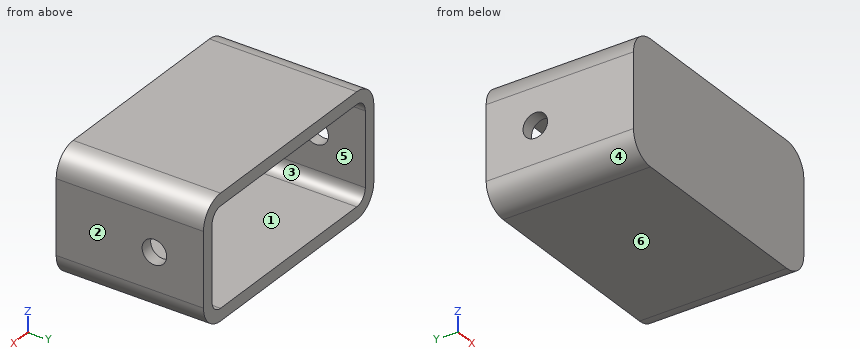
from build123d import *

# Parameters (mm, degrees)
SKETCH1_W           = 100
SKETCH1_H           = 60
BOSS_EXTRUDE1_DEPTH = 50
FILLET1_R           = 10
SHELL1_T            = -5
SKETCH2_R           = 5
CUT_EXTRUDE1_DEPTH  = 101


with BuildPart() as part:
    # Sketch1 → Boss-Extrude1 (new body)
    with BuildSketch(Plane.XY):
        with Locations((50, 30)):
            Rectangle(SKETCH1_W, SKETCH1_H)
    extrude(amount=BOSS_EXTRUDE1_DEPTH)

    # Fillet1
    fillet1_edges = [part.edges().sort_by_distance(p)[0] for p in [
        (100, 30, 50),
        (0, 30, 50),
        (100, 30, 0),
        (0, 30, 0),
    ]]
    fillet(fillet1_edges, radius=FILLET1_R)

    # Shell1
    shell1_openings = [part.faces().sort_by_distance(p)[0] for p in [
        (50, 60, 25),
    ]]
    offset(amount=SHELL1_T, openings=shell1_openings, kind=Kind.INTERSECTION)

    # Sketch2 → Cut-Extrude1 (cut, through all)
    with BuildSketch(Plane(origin=(100, 0, 0), x_dir=(0, 0, -1), z_dir=(1, 0, 0))):
        with Locations((-25, 40)):
            Circle(SKETCH2_R)
    extrude(amount=-CUT_EXTRUDE1_DEPTH, mode=Mode.SUBTRACT)


solid = part.part
Read the model definition and answer for the solid it produces. Units are mm, in the model's axes. Face numbers are marked on the shaded views. A direction names the side the tool comes from. Round coordinates to 2 decimals unless told otherwise and drop trailing zeros. Loops run counter-clockwise (first coordinate to the right, second up) from the corner with the lowest first, then second, coordinate; pieces in that order, holes last. Notation, with made-up numbers: (78, 70.5) - (98, 70.5) arc R20 ccw to (98, 98.5) - close; hole circle Ø3 at (44, 70). An arc over 180 degrees is marked (long way). One line per question, with ' | ' between items. Start each with the question number.
Q1. Find the intervals of material crossed by L1, parallel to Y at x = 98, z = 25; L2, parallel to Z at x = 45.5, y = 14.5; L3, parallel to X at y = 36.5, z = 34, in increasing order.
Q2. Section C-C on z = 18 is taken. Give the vertices of the cut face in (x, y).
Q3. For the marked faces 1 and 2, determine the directions among +Z, -Z, +X, -X, +Y, -Y from which every point of the face is accessible in a straight line to the end or side of a thin tool.
Q4. Flat-ended cylindrical pins translate along their axes: pin 1 (12 mm diameter, centred on x = 62.5, z = 18, fed in from +Y); pin 2 (6 mm diameter, centred on y = 40, z = 25, fed in from +X). Find the tip coordinate at first contact, or state that the pin passes through.
Q5. For a pull along X with two mould halves and no side action, classify the marked faces 3, 4, 5 and 6 as +X half, -X half, draft (parallel to the pull), parting line (faces both ways), or undercut.
Q6. Section D-D on y = 12 is taken. Give the vertices of the cut face in (x, z).
Q7. Section B-B on z = 25 is taken. Give the vertices of the cut face in (x, y).
Q8. Section A-A on y = 40 is taken. Give the vertices of the cut face in (x, z).
Established:
1) L1: 0 to 35, 45 to 60 | L2: 0 to 5, 45 to 50 | L3: 0 to 5, 95 to 100
2) outline: (0, 0) - (100, 0) - (100, 60) - (95, 60) - (95, 5) - (5, 5) - (5, 60) - (0, 60) - close
3) face 1: +Y | face 2: +Z, -Z, +X, +Y, -Y
4) pin 1: y = 5 | pin 2: through
5) face 3: undercut | face 4: -X half | face 5: undercut | face 6: draft
6) outline: (0, 10) arc R10 ccw to (10, 0) - (90, 0) arc R10 ccw to (100, 10) - (100, 40) arc R10 ccw to (90, 50) - (10, 50) arc R10 ccw to (0, 40) - close; hole (5, 10) arc R5 ccw to (10, 5) - (90, 5) arc R5 ccw to (95, 10) - (95, 40) arc R5 ccw to (90, 45) - (10, 45) arc R5 ccw to (5, 40) - close
7) outline: (0, 0) - (100, 0) - (100, 35) - (95, 35) - (95, 5) - (5, 5) - (5, 35) - (0, 35) - close; (0, 45) - (5, 45) - (5, 60) - (0, 60) - close; (95, 45) - (100, 45) - (100, 60) - (95, 60) - close
8) outline: (0, 10) arc R10 ccw to (10, 0) - (90, 0) arc R10 ccw to (100, 10) - (100, 20) - (95, 20) - (95, 10) arc R5 cw to (90, 5) - (10, 5) arc R5 cw to (5, 10) - (5, 20) - (0, 20) - close; (0, 30) - (5, 30) - (5, 40) arc R5 cw to (10, 45) - (90, 45) arc R5 cw to (95, 40) - (95, 30) - (100, 30) - (100, 40) arc R10 ccw to (90, 50) - (10, 50) arc R10 ccw to (0, 40) - close
